Autodesk Inventor part; units mm, degrees
ref_plane "Arbeitsebene1" through (0, 0, 10) normal (0, 0, 1) x (1, 0, 0)
ref_plane "YZ Plane" through (0, 0, 0) normal (1, 0, 0) x (0, 1, 0)
ref_plane "XZ Plane" through (0, 0, 0) normal (0, 1, 0) x (-1, 0, 0)
ref_plane "Arbeitsebene1" through (0, 0, 10) normal (0, 0, 1) x (1, 0, 0)
sketch "Skizze1" plane through (0, 0, 0) normal (0, 0, 1) x (1, 0, 0)
  line L0 (-27.5, 25.5) -> (27.5, 25.5)
  line L1 (32.5, 20.5) -> (32.5, -20.5)
  line L2 (27.5, -25.5) -> (-27.5, -25.5)
  line L3 (-32.5, -20.5) -> (-32.5, 20.5)
  line L4 (-32.5, 0) -> (32.5, 0) construction
  line L5 (0, 25.5) -> (0, -25.5) construction
  line L6 (-32.5, 20.5) -> (-27.5, 25.5)
  line L7 (32.5, 20.5) -> (27.5, 25.5)
  line L8 (-32.5, -20.5) -> (-27.5, -25.5)
  line L9 (32.5, -20.5) -> (27.5, -25.5)
  point P0 (0, 0)
  point P1 (0, 0)
  dimension "d0" = 65
  dimension "d3" = 5
  dimension "d4" = 51
  dimension "d28" = 5
sketch "Skizze2" plane through (0, 0, 10) normal (0, 0, 1) x (1, 0, 0)
  line L0 (-48, 29) -> (48, 29)
  line L1 (53, 24) -> (53, -24)
  line L2 (48, -29) -> (-48, -29)
  line L3 (-53, -24) -> (-53, 24)
  line L4 (-53, 0) -> (53, 0) construction
  line L5 (0, 29) -> (0, -29) construction
  line L6 (-53, 24) -> (-48, 29)
  line L7 (53, 24) -> (48, 29)
  line L8 (-53, -24) -> (-48, -29)
  line L9 (53, -24) -> (48, -29)
  point P0 (0, 0)
  point P1 (0, 0)
  dimension "d6" = 58
  dimension "d8" = 45
  dimension "d9" = 5
  dimension "d10" = 106
loft "Erhebung1" add profiles "Skizze1", "Skizze2"
sketch "Skizze3" plane through (27.5, 25.5, 0) normal (0, 0, -1) x (-1, 0, 0)
  line L0 (14, -51) -> (41, -51)
  line L1 (41, -51) -> (41, -9)
  line L2 (41, -9) -> (14, -9)
  line L3 (14, -9) -> (14, -51)
  line L4 (55, -51) -> (0, -51)
  point P0 (27.5, -25.5)
  point P1 (27.5, -51)
  dimension "d15" = 27
  dimension "d16" = 42
extrude "Extrusion1" add sketch "Skizze3" along normal blind 13
sketch "Skizze4" plane through (-13.5, -25.5, 0) normal (0, -1, 0) x (1, 0, 0)
  line L0 (13.5, 0) -> (13.5, -13) construction
  line L1 (27, -13) -> (0, -13) construction
  circle A0 centre (13.5, -6.5) radius 2.15
  line L2 (27, 0) -> (27, -13)
  line L3 (27, -13) -> (22.5, 0)
  line L4 (0, 0) -> (27, 0)
  line L5 (0, -13) -> (4.5, 0)
  line L6 (0, 0) -> (27, 0)
  line L7 (0, 0) -> (0, -13)
  line L8 (27, -13) -> (0, -13)
  line L9 (27, 0) -> (27, -13)
  line L10 (26.6825, -13) -> (22.1825, 0)
  line L11 (4.8175, 0) -> (0.3175, -13)
  line L12 (0.1038, -12.7) -> (26.8962, -12.7)
  point P0 (26.5787, -12.7)
  point P1 (0.4213, -12.7)
  point P2 (22.1825, 0)
  dimension "d19" = 18
  dimension "d20" = 4.3
  dimension "d29" = 27
  dimension "d30" = 13
  dimension "d31" = 0.3
  dimension "d32" = 0.3
  dimension "d33" = 0.3
extrude "Extrusion2" cut sketch "Skizze4" against normal through all contours A0 | L2 L3 L4 | L8 L10 L12 L3 | L3 L12 L10 L4 | L8 L11 L12 L10 | L8 L5 L12 L11 | L11 L12 L5 L4 | L7 L4 L5
sketch "Skizze5" plane through (27.5, 25.5, 0) normal (0, 0, -1) x (-1, 0, 0)
  line L0 (2.5, -5.5) -> (52.5, -5.5)
  line L1 (52.5, -5.5) -> (52.5, -45.5)
  line L2 (52.5, -45.5) -> (2.5, -45.5)
  line L3 (2.5, -45.5) -> (2.5, -5.5)
  line L4 (2.5, -5.5) -> (52.5, -45.5) construction
  line L5 (52.5, -5.5) -> (2.5, -45.5) construction
  circle A0 centre (2.5, -5.5) radius 1.75
  circle A1 centre (52.5, -5.5) radius 1.75
  circle A2 centre (2.5, -45.5) radius 1.75
  circle A3 centre (52.5, -45.5) radius 1.75
  point P0 (27.5, -25.5)
  point P1 (27.5, -25.5)
  point P2 (27.5, -25.5)
  dimension "d23" = 50
  dimension "d24" = 40
  dimension "d25" = 3.5
extrude "Extrusion3" cut sketch "Skizze5" against normal through all contours L3 A0 L0 | L0 A0 L3 | A1 L1 L0 | L0 L1 A1 | A2 L2 L3 | L3 L2 A2 | A3 L2 L1 | L1 L2 A3
sketch "Skizze6" plane through (27.5, 25.5, 0) normal (0, 0, -1) x (-1, 0, 0)
  circle A0 centre (2.5, -5.5) radius 1.75
  line L0 (-0.9641, -5.5) -> (0.7679, -2.5)
  line L1 (0.7679, -2.5) -> (4.2321, -2.5)
  line L2 (4.2321, -2.5) -> (5.9641, -5.5)
  line L3 (5.9641, -5.5) -> (4.2321, -8.5)
  line L4 (4.2321, -8.5) -> (0.7679, -8.5)
  line L5 (0.7679, -8.5) -> (-0.9641, -5.5)
  line L6 (0, 0) -> (55, 0)
  line L7 (27.5, 0) -> (27.5, -51) construction
  line L8 (36.1825, -51) -> (18.8175, -51) construction
  line L9 (-5, -46) -> (-5, -5) construction
  line L10 (-5, -25.5) -> (60, -25.5) construction
  line L11 (60, -5) -> (60, -46) construction
  circle A1 centre (52.5, -5.5) radius 1.75
  line L12 (55.9641, -5.5) -> (54.2321, -2.5)
  line L13 (54.2321, -2.5) -> (50.7679, -2.5)
  line L14 (50.7679, -2.5) -> (49.0359, -5.5)
  line L15 (49.0359, -5.5) -> (50.7679, -8.5)
  line L16 (50.7679, -8.5) -> (54.2321, -8.5)
  line L17 (54.2321, -8.5) -> (55.9641, -5.5)
  line L18 (55, 0) -> (0, 0)
  circle A2 centre (2.5, -45.5) radius 1.75
  line L19 (-0.9641, -45.5) -> (0.7679, -48.5)
  line L20 (0.7679, -48.5) -> (4.2321, -48.5)
  line L21 (4.2321, -48.5) -> (5.9641, -45.5)
  line L22 (5.9641, -45.5) -> (4.2321, -42.5)
  line L23 (4.2321, -42.5) -> (0.7679, -42.5)
  line L24 (0.7679, -42.5) -> (-0.9641, -45.5)
  line L25 (54.2321, -48.5) -> (50.7679, -48.5)
  line L26 (55.9641, -45.5) -> (54.2321, -48.5)
  circle A3 centre (52.5, -45.5) radius 1.75
  line L27 (50.7679, -48.5) -> (49.0359, -45.5)
  line L28 (54.2321, -42.5) -> (55.9641, -45.5)
  line L29 (50.7679, -42.5) -> (54.2321, -42.5)
  line L30 (49.0359, -45.5) -> (50.7679, -42.5)
  point P0 (27.5, -25.5)
  dimension "d34" = 6
extrude "Extrusion4" cut sketch "Skizze6" against normal blind 6 contours A0 | L0 L1 L2 L3 L4 L5 | A1 | L17 L16 L15 L14 L13 L12 | A2 | L24 L23 L22 L21 L20 L19 | L25 L27 L30 L29 L28 L26 | A3
sketch "Skizze7" plane through (-8.6825, 16.5, 0) normal (0, 1, 0) x (1, 0, 0)
  circle A0 centre (8.6825, 6.5) radius 2.15
  line L0 (6.5752, 10.15) -> (10.7899, 10.15)
  line L1 (10.7899, 10.15) -> (12.8972, 6.5)
  line L2 (12.8972, 6.5) -> (10.7899, 2.85)
  line L3 (10.7899, 2.85) -> (6.5752, 2.85)
  line L4 (6.5752, 2.85) -> (4.4679, 6.5)
  line L5 (4.4679, 6.5) -> (6.5752, 10.15)
  line L6 (21.7612, 12.7) -> (-4.3962, 12.7)
  line L7 (4.4679, 6.5) -> (4.4679, 12.7)
  line L8 (12.8972, 6.5) -> (12.8972, 12.7)
  line L9 (-4.3962, 12.7) -> (21.7612, 12.7)
  line L10 (4.4679, 12.7) -> (12.8972, 12.7)
  point P0 (8.6825, 0)
  dimension "d37" = 7.3
extrude "Extrusion5" cut sketch "Skizze7" against normal blind 10
extrude "Extrusion6" add sketch "Skizze7" against normal blind 6.5
equation "\"d32\" = d31"
equation "\"d33\" = d32"
properties part number "5,1_3D-Druck"
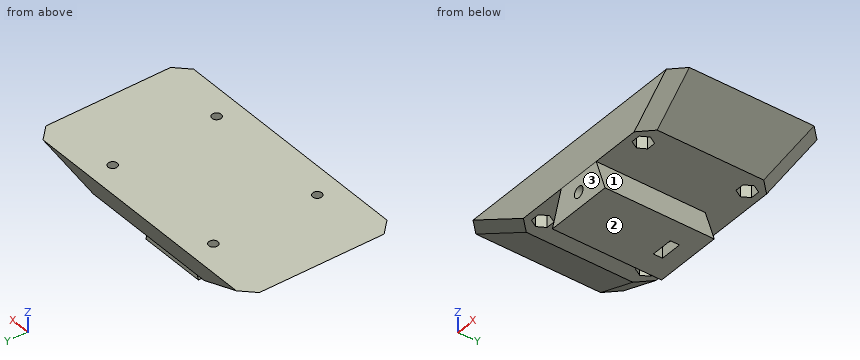
CAD build for the part. Positions are in the model's coordinates, mm. Face numbers are marked on the shaded views. Coordinates: 2 decimals unless noted, no trailing zeros. Order: outer loops, then holes, each group sorted by start corner. A loop starts at its lowest first (then second) coordinate and runs counter-clockwise, first axis right, second up. Notation, with made-up numbers: (64, 19.25) - (86, 19.25) arc R9 cw to (86, 29.25) - close; hole circle Ø9 at (76.25, 38). An arc over 180 degrees is marked (long way). Use a Markdown table: item, result. Add a question column.
(1) Saw through at B-B (x = -25). Count the separate pieces of the cut face and the enclosed holes in it, then the cut area to 3 significant figures.
(2) Pull direction Z, two halves, no side cores. Call the marked faces 1, 2 and 3: +Z half, -Z half, draft (parallel to the pull), parting line (faces both ways), or undercut.
(3) Saw through at A-A (z = -7.5). Give the cut face in (x, y), then the cut area to 3 significant figures.
(4) Flat gauge pins, fed straight in: pin 1 (1 mm diameter, centred on x = 25, z = 2, fed in from +Y) (3 decimals); pin 2 (4 mm diameter, centred on x = 29.5, y = 8, fed in from -Z); pin 3 (3 mm diameter, centred on x = 25.5, z = 2.5, fed in from -Y). Where does each tip first touch, or does it go through?
(5) Drill centre lines: line 1 along Y through (x, z) = (-25, 8.5) (3 decimals); line 2 along Z through (x, y) = (0, -11); line 3 along Y through (x, z) = (-25, 8.85). Where is each one in solid material? Low to high. Write a range as [from, to].
Solved:
| question | item | result |
|---|---|---|
| 1 | separate pieces | 3 |
| 1 | enclosed holes | 0 |
| 1 | area | 445 mm² |
| 2 | face 1 | undercut |
| 2 | face 2 | -Z half |
| 2 | face 3 | draft |
| 3 | outline | (-11.28, -25.5) - (-1.9, -25.5) - (-1.9, 6.5) - (-4.21, 6.5) - (-4.21, 10) - (-1.9, 10) - (-1.9, 16.5) - (-11.28, 16.5) - close; (1.9, -25.5) - (11.28, -25.5) - (11.28, 16.5) - (1.9, 16.5) - (1.9, 10) - (4.21, 10) - (4.21, 6.5) - (1.9, 6.5) - close |
| 3 | area | 771 mm² |
| 4 | pin 1 | stops at y = 26.375 |
| 4 | pin 2 | stops at z = 0 |
| 4 | pin 3 | stops at y = -26.9 |
| 5 | line 1 | y = [-28.475, -21.75], [-18.25, 18.25], [21.75, 28.475] |
| 5 | line 2 | z = [-12.7, -8.65], [-4.35, 10] |
| 5 | line 3 | y = [-28.6, -21.75], [-18.25, 18.25], [21.75, 28.6] |
